CAD build for the part. Positions are in the model's coordinates, mm. Round coordinates to 2 decimals unless told otherwise and drop trailing zeros. Loops run counter-clockwise (first coordinate to the right, second up) from the corner with the lowest first, then second, coordinate; pieces in that order, holes last. Notation, with made-up numbers: M 57.5,70 L 83.5,70 A20 cw 83.5,79 Z; hole C 30.25,-0.5 d8. An arc over 180 degrees is marked long. Use a Markdown table: item, result. Add a question column.
(1) Band-saw the part on C-C, the plane x = 309.5. Write the cut outline in (y, z) (3 decimals).
(2) Band-saw the part on B-B, the plane z = 0.75. Write the cut outline in (x, y) (3 decimals), and give its area (3 significant figures).
(3) Two-plate mould, pull along X, no slides. Class faces 1 (the face through (326.06, 211.04, 1.61)), 2 (the face through (180, 121, 3.175)): released by +X, released by -X, zero draft, split by the parting line, or undercut.
(4) Band-saw the part on A-A, the plane y = 215.9. Write the cut outline in (x, z) (3 decimals).
(5) Wall check: L1, parallel to Y at x = 315, z = 2.7; L2, parallel to Y at x = 45.5, z = 2.85; L3, parallel to Y at x = 322, z = 1.45. Give the ranges that are in metal, low to high.
(6) Band-saw the part on D-D, the plane y = 99. Write the cut outline in (x, z) (3 decimals), and give its area (3 significant figures).
(7) Flat gauge pins, fed straight in: P1, Ø20.5, axis at x = 314.325, y = 215.9, coming from the +Z side; P2, Ø1.5, axis at y = 106.5, z = 2, coming from the +X side (3 decimals); P3, Ø1.6, axis at x = 354, z = 1.5, coming from the -Y side; P4, Ø1, axis at x = 2, z = 1, coming from the -Y side. Where does each tip first touch, or does it go through?
from build123d import *

# Parameters (mm, degrees)
BOSS_EXTRUDE1_DEPTH = 3.175
SKETCH2_R           = 12.7
CUT_EXTRUDE1_DEPTH  = 4.175


with BuildPart() as part:
    # Sketch1 → Boss-Extrude1 (new body)
    with BuildSketch(Plane.XY):
        with BuildLine():
            Line((0, 228.6), (0, 250.825))
            Line((0, 250.825), (0, 254))
            Line((0, 254), (3.175, 254))
            Line((3.175, 254), (3.175, 250.825))
            Line((3.175, 250.825), (25.4, 250.825))
            Line((25.4, 250.825), (25.4, 254))
            Line((25.4, 254), (330.2, 254))
            Line((330.2, 254), (330.2, 250.825))
            Line((330.2, 250.825), (352.425, 250.825))
            Line((352.425, 250.825), (352.425, 254))
            Line((352.425, 254), (355.6, 254))
            Line((355.6, 254), (355.6, 250.825))
            Line((355.6, 250.825), (355.6, 228.6))
            Line((355.6, 228.6), (352.425, 228.6))
            Line((352.425, 228.6), (352.425, 25.4))
            Line((352.425, 25.4), (355.6, 25.4))
            Line((355.6, 25.4), (355.6, 0))
            ThreePointArc((355.6, 0), (339.725, -15.875), (323.85, 0))
            Line((323.85, 0), (31.75, 0))
            ThreePointArc((31.75, 0), (15.875, -15.875), (0, 0))
            Line((0, 0), (0, 25.4))
            Line((0, 25.4), (3.175, 25.4))
            Line((3.175, 25.4), (3.175, 228.6))
            Line((3.175, 228.6), (0, 228.6))
        make_face()
    extrude(amount=BOSS_EXTRUDE1_DEPTH)

    # Sketch2 → Cut-Extrude1 (cut, through all)
    with BuildSketch(Plane.XY.offset(3.175)):
        with Locations((314.325, 215.9)):
            Circle(SKETCH2_R)
    extrude(amount=-CUT_EXTRUDE1_DEPTH, mode=Mode.SUBTRACT)


solid = part.part
Return value:
| question | item | result |
|---|---|---|
| 1 | outline | M 0,0 L 204.152,0 L 204.152,3.175 L 0,3.175 Z; M 227.648,0 L 254,0 L 254,3.175 L 227.648,3.175 Z |
| 2 | outline | M 0,0 A15.875 ccw 31.75,0 L 323.85,0 A15.875 ccw 355.6,0 L 355.6,25.4 L 352.425,25.4 L 352.425,228.6 L 355.6,228.6 L 355.6,254 L 352.425,254 L 352.425,250.825 L 330.2,250.825 L 330.2,254 L 25.4,254 L 25.4,250.825 L 3.175,250.825 L 3.175,254 L 0,254 L 0,228.6 L 3.175,228.6 L 3.175,25.4 L 0,25.4 Z; hole C 314.325,215.9 d25.4 |
| 2 | area | 89,200 mm^2 |
| 3 | face 1 | undercut |
| 3 | face 2 | zero draft |
| 4 | outline | M 3.175,0 L 301.625,0 L 301.625,3.175 L 3.175,3.175 Z; M 327.025,0 L 352.425,0 L 352.425,3.175 L 327.025,3.175 Z |
| 5 | L1 | 0 to 203.22, 228.58 to 254 |
| 5 | L2 | 0 to 254 |
| 5 | L3 | 0 to 205.78, 226.02 to 254 |
| 6 | outline | M 3.175,0 L 352.425,0 L 352.425,3.175 L 3.175,3.175 Z |
| 6 | area | 1,110 mm^2 |
| 7 | P1 | through |
| 7 | P2 | x = 352.425 |
| 7 | P3 | y = -8.39 |
| 7 | P4 | y = -8.55 |
